The figure shows three views and two pictorial views of one solid part (mm, origin at its lowest corner). Answer the questions. A direction names the side the tool comes from. Coordinates: 2 decimals unless noted, no trailing zeros. Order: outer loops, then holes, each group sorted by start corner. A loop starts at its lowest first (then second) coordinate and runs counter-clockwise, first axis right, second up. Notation, with made-up numbers: (5.25, 84.25) - (40.25, 84.25) arc R17 cw to (40.25, 92.25) - close; hole circle Ø2 at (5.5, 20). An arc over 180 degrees is marked (long way). Use one line per item in the form item = value. Start each with the question number.
Item 1: Section D-D, the plane y = 24 is taken. Write down the section's boundary in (x, z).
Item 2: Section C-C, the plane z = 16.35 is taken. Write down the section's boundary in (x, y), and give its area (3 significant figures).
Item 3: The mould has two halves that part along Z. Classify the marked faces 1, 2, 3 and 4: released by +Z, released by -Z, zero draft, split by the parting line, or undercut.
Item 4: Section A-A, the plane y = 35 is taken. Write down the section's boundary in (x, z).
Item 5: Consider line 1 along Y through (x, z) = (2.5, 16.35); line 2 along Z through (x, y) = (3, 3); line 3 along Y through (x, z) = (3, 30). Determine where each line is inside the solid, lowest interval first. Write a range as [from, to].
Item 6: Each of these flat-tipped pins is pushed along its axis until it touches: pin 1 Ø1.3 at (x, z) = (3.5, 28.5) entering from +Y; pin 2 Ø1.3 at (x, z) = (3.5, 27.5) entering from -Y; pin 3 Ø2.5 at (x, y) = (2.5, 3.5) entering from -Z. Where does it stop, or does it pass through?
Item 7: A tool of negligible diameter and unlimited length cuts with its end or side. For the marked faces 5, 6, 7 and 8, from which of +Z, -Z, +X, -X, +Y, -Y can it reach the whole face along a straight path? Write none if from no direction.
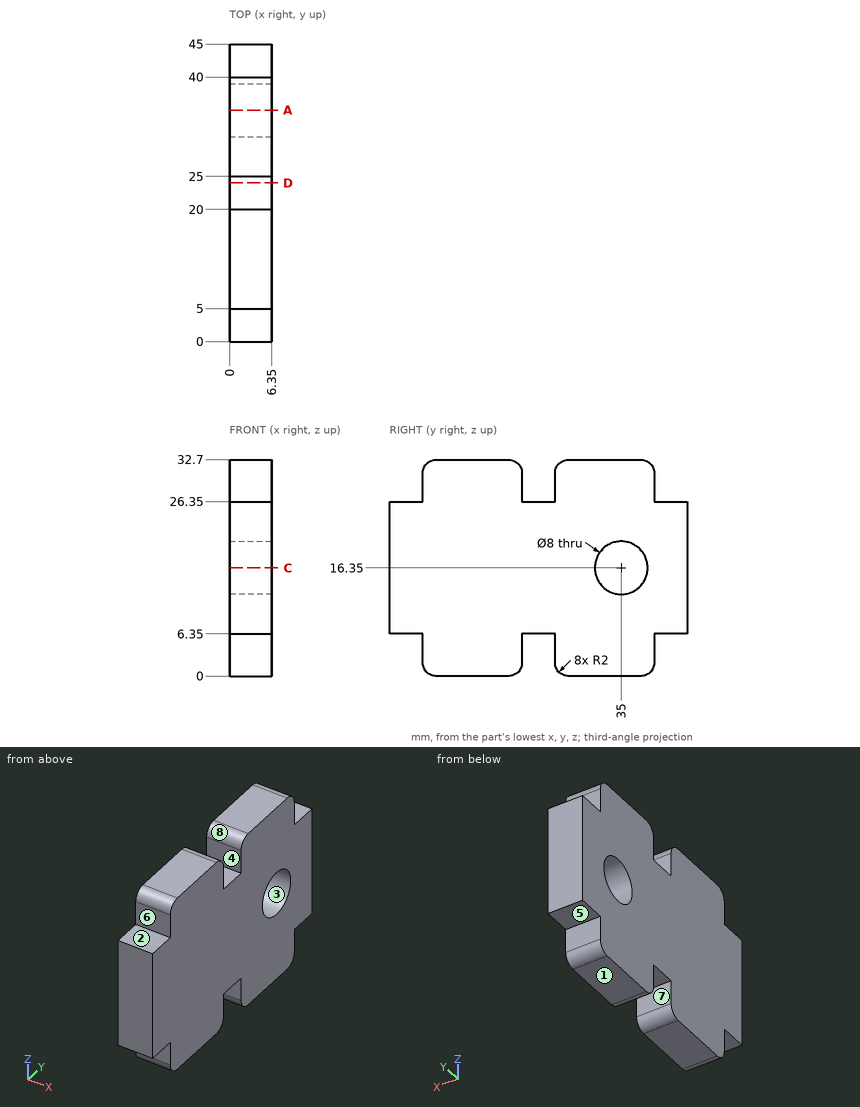
Response:
q1.outline = (0, 6.35) - (6.35, 6.35) - (6.35, 26.35) - (0, 26.35) - close
q2.outline = (0, 0) - (6.35, 0) - (6.35, 31) - (0, 31) - close; (0, 39) - (6.35, 39) - (6.35, 45) - (0, 45) - close
q2.area = 235 mm2
q3.face_1 = released by -Z
q3.face_2 = released by +Z
q3.face_3 = undercut
q3.face_4 = zero draft
q4.outline = (0, 0) - (6.35, 0) - (6.35, 12.35) - (0, 12.35) - close; (0, 20.35) - (6.35, 20.35) - (6.35, 32.7) - (0, 32.7) - close
q5.line_1 = [0, 31], [39, 45]
q5.line_2 = [6.35, 26.35]
q5.line_3 = [5, 20], [25, 40]
q6.pin_1 = 40
q6.pin_2 = 5
q6.pin_3 = 6.35
q7.face_5 = -Z, +X, -X, +Y
q7.face_6 = +Z, +X, -X, -Y
q7.face_7 = -Z, +X, -X
q7.face_8 = +Z, +X, -X
